```python
from build123d import *

# Parameters (mm, degrees)
SKETCH1_R           = 4.7625
EXTRUDE1_DEPTH      = 38.1
CHAMFER1_SIZE       = 0.714375
EXTRUDE2_DEPTH      = 39.690732902
EXTRUDE2_DEPTH_BACK = 39.690732902
SKETCH3_W           = 2.38125
SKETCH3_H           = 1.190625


with BuildPart() as part:
    # Sketch1 → Extrude1 (new, symmetric)
    with BuildSketch(Plane.XY):
        with Locations(Location((0, 0, 0), (0, 0, 180))):
            Circle(SKETCH1_R)
    extrude(amount=EXTRUDE1_DEPTH, both=True)

    # Chamfer1
    chamfer1_edges = [part.edges().sort_by_distance(p)[0] for p in [
        (4.7625, 0, -38.1),
        (4.7625, 0, 38.1),
    ]]
    chamfer(chamfer1_edges, length=CHAMFER1_SIZE)

    # Sketch3 → Extrude2 (cut, two sides: drawn at the far end of the back side and taken through both)
    with BuildSketch(Plane.XY.offset(-EXTRUDE2_DEPTH_BACK)):
        with Locations((0, 4.1671875)):
            Rectangle(SKETCH3_W, SKETCH3_H)
    extrude(amount=EXTRUDE2_DEPTH + EXTRUDE2_DEPTH_BACK, mode=Mode.SUBTRACT)


solid = part.part
```
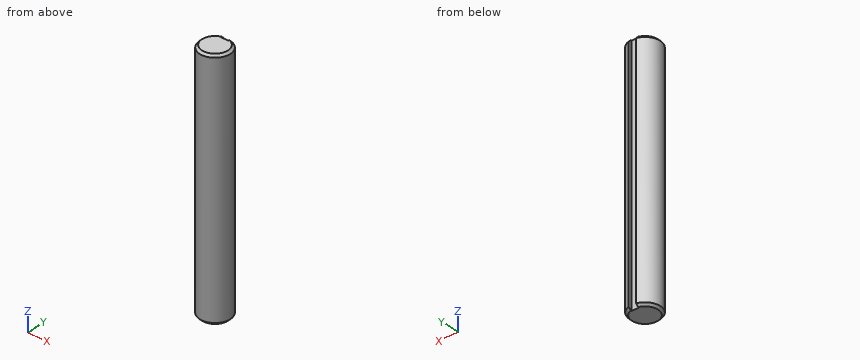
CAD build for the part. Positions are in the model's coordinates, mm. Round coordinates to 2 decimals unless told otherwise and drop trailing zeros. Loops run counter-clockwise (first coordinate to the right, second up) from the corner with the lowest first, then second, coordinate; pieces in that order, holes last. Notation, with made-up numbers: M 65,-25.75 L 112,-25.75 A24 cw 112,0.25 Z; hole C 40.25,2.5 d7. An arc over 180 degrees is marked long. Return JSON: item names as keys, results as strings. Group by question number.
(1) Saw through at B-B, the plane z = 7.5. List the corners of the cut face in (x, y) (1 decimal), and give its area (3 significant figures).
(2) Saw through at A-A, the plane x = 0. List the corners of the cut face in (y, z).
(3) Wall check: probe 1 along X at (y, z) = (0.25, 1.5); probe 2 along X at (y, z) = (2.5, 17.5); probe 3 along Z at (x, y) = (-3.75, -1.75). Give the ranges that are in metal, low to high. Write a range as [from, to].
(4) Drop flat-ended pins along their axis: P1, Ø1.1, axis at y = 4, z = 9.5, coming from the +X side; P2, Ø1.5, axis at y = -2.5, z = -12, coming from the -X side. Give the stop position or say it passes through.
Answer list:
{
 "1": {"outline": "M -1.2,3.6 L -1.2,4.6 A4.8 ccw long 1.2,4.6 L 1.2,3.6 Z", "area": "68.5 mm2"},
 "2": {"outline": "M -4.76,-37.39 L -4.05,-38.1 L 3.57,-38.1 L 3.57,38.1 L -4.05,38.1 L -4.76,37.39 Z"},
 "3": {"probe 1": "[-4.76, 4.76]", "probe 2": "[-4.05, 4.05]", "probe 3": "[-38.01, 38.01]"},
 "4": {"P1": "x = 3.28", "P2": "x = -4.43"}
}
